```python
from build123d import *

# Parameters (mm, degrees)
CYLINDER004_R     = 7
CYLINDER004_DEPTH = 1
BOX003_W          = 12
BOX003_H          = 21
BOX003_DEPTH      = 19.6
BOX002_W          = 5.7
BOX002_H          = 7.6
BOX002_DEPTH      = 3
BOX001_W          = 35.56
BOX001_H          = 17.78
BOX001_DEPTH      = 10
BOX004_W          = 13.749
BOX004_H          = 12
BOX004_DEPTH      = 4
BOX005_W          = 11.3259
BOX005_H          = 12
BOX005_DEPTH      = 4
CYLINDER005_R     = 3.25
CYLINDER005_DEPTH = 3.5
BOX006_W          = 14.4
BOX006_H          = 9
BOX006_DEPTH      = 11
CYLINDER007_R     = 2
CYLINDER007_DEPTH = 5
CYLINDER006_R     = 2
CYLINDER006_DEPTH = 5
CYLINDER009_R     = 2.5
CYLINDER009_DEPTH = 5
CYLINDER008_R     = 10.9
CYLINDER008_DEPTH = 2.6
BOX007_W          = 18.3
BOX007_H          = 21.8
BOX007_DEPTH      = 24.8
CYLINDER010_R     = 2.5
CYLINDER010_DEPTH = 5
CYLINDER001_R     = 1.8
CYLINDER001_DEPTH = 1.8
CYLINDER002_R     = 1.8
CYLINDER002_DEPTH = 1.8
CYLINDER003_R     = 1.8
CYLINDER003_DEPTH = 1.8
CYLINDER_R        = 1.8
CYLINDER_DEPTH    = 1.8
BOX_W             = 76.2
BOX_H             = 68.58
BOX_DEPTH         = 1.8
FILLET_R          = 3.81
CYLINDER015_R     = 2
CYLINDER015_DEPTH = 5
CYLINDER011_R     = 2
CYLINDER011_DEPTH = 5
CYLINDER012_R     = 2.5
CYLINDER012_DEPTH = 5
CYLINDER014_R     = 10.9
CYLINDER014_DEPTH = 2.6
BOX008_W          = 18.3
BOX008_H          = 21.8
BOX008_DEPTH      = 24.8
CYLINDER013_R     = 2.5
CYLINDER013_DEPTH = 5


with BuildPart() as cylinder004:
    # Cylinder004 → Cylinder004 (new body)
    with BuildSketch(Plane(origin=(0, 50.8, 11.4), x_dir=(0, 0, -1), z_dir=(1, 0, 0))):
        Circle(CYLINDER004_R)
    extrude(amount=CYLINDER004_DEPTH)


with BuildPart() as midi:
    # Box003 → Box003 (new body)
    with BuildSketch(Plane(origin=(0, 40.3, 1.8), x_dir=(1, 0, 0), z_dir=(0, 0, 1))):
        with Locations((6, 10.5)):
            Rectangle(BOX003_W, BOX003_H)
    extrude(amount=BOX003_DEPTH)

    # Cut001: cut Cylinder004
    add(cylinder004.part, mode=Mode.SUBTRACT)


with BuildPart() as cube002:
    # Box002 → Box002 (new body)
    with BuildSketch(Plane(origin=(0, 16.53, 11.8), x_dir=(1, 0, 0), z_dir=(0, 0, 1))):
        with Locations((2.85, 3.8)):
            Rectangle(BOX002_W, BOX002_H)
    extrude(amount=BOX002_DEPTH)


with BuildPart() as obj1:
    # Box001 → Box001 (new body)
    with BuildSketch(Plane(origin=(0, 11.44, 1.8), x_dir=(1, 0, 0), z_dir=(0, 0, 1))):
        with Locations((17.78, 8.89)):
            Rectangle(BOX001_W, BOX001_H)
    extrude(amount=BOX001_DEPTH)

    # Fusion001: union Cube002
    add(cube002.part)


with BuildPart() as obj2:
    # Box004 → Box004 (new body)
    with BuildSketch(Plane(origin=(38.8544, 0, 1.8), x_dir=(1, 0, 0), z_dir=(0, 0, 1))):
        with Locations((6.8745, 6)):
            Rectangle(BOX004_W, BOX004_H)
    extrude(amount=BOX004_DEPTH)


with BuildPart() as obj3:
    # Box005 → Box005 (new body)
    with BuildSketch(Plane(origin=(40.005, 56.58, 1.8), x_dir=(1, 0, 0), z_dir=(0, 0, 1))):
        with Locations((5.66295, 6)):
            Rectangle(BOX005_W, BOX005_H)
    extrude(amount=BOX005_DEPTH)


with BuildPart() as cylinder005:
    # Cylinder005 → Cylinder005 (new body)
    with BuildSketch(Plane(origin=(10.9, 4.5, 8.3), x_dir=(0, 0, -1), z_dir=(1, 0, 0))):
        Circle(CYLINDER005_R)
    extrude(amount=CYLINDER005_DEPTH)


with BuildPart() as dc_jack:
    # Box006 → Box006 (new body)
    with BuildSketch(Plane.XY.offset(1.8)):
        with Locations((7.2, 4.5)):
            Rectangle(BOX006_W, BOX006_H)
    extrude(amount=BOX006_DEPTH)

    # Cut002: cut Cylinder005
    add(cylinder005.part, mode=Mode.SUBTRACT)


with BuildPart() as dc_jack_1:
    # Cut002 placement: moved
    add(dc_jack.part.moved(Location((64.4, 1.85, 0))))


with BuildPart() as cylinder007:
    # Cylinder007 → Cylinder007 (new body)
    with BuildSketch(Plane(origin=(13.3, 20.8, 2.5), x_dir=(0, 0, -1), z_dir=(1, 0, 0))):
        Circle(CYLINDER007_R)
    extrude(amount=CYLINDER007_DEPTH)


with BuildPart() as fusion003:
    # Cylinder006 → Cylinder006 (new body)
    with BuildSketch(Plane(origin=(13.3, 1, 22.3), x_dir=(0, 0, -1), z_dir=(1, 0, 0))):
        Circle(CYLINDER006_R)
    extrude(amount=CYLINDER006_DEPTH)

    # Fusion003: union Cylinder007
    add(cylinder007.part)


with BuildPart() as cylinder009:
    # Cylinder009 → Cylinder009 (new body)
    with BuildSketch(Plane(origin=(13.3, 1, 22.3), x_dir=(0, 0, -1), z_dir=(1, 0, 0))):
        Circle(CYLINDER009_R)
    extrude(amount=CYLINDER009_DEPTH)


with BuildPart() as cylinder008:
    # Cylinder008 → Cylinder008 (new body)
    with BuildSketch(Plane(origin=(18.3, 10.9, 12.4), x_dir=(0, 0, -1), z_dir=(1, 0, 0))):
        Circle(CYLINDER008_R)
    extrude(amount=CYLINDER008_DEPTH)


with BuildPart() as cube005:
    # Box007 → Box007 (new body)
    with BuildSketch(Plane.XY):
        with Locations((9.15, 10.9)):
            Rectangle(BOX007_W, BOX007_H)
    extrude(amount=BOX007_DEPTH)


with BuildPart() as obj4:
    # Cylinder010 → Cylinder010 (new body)
    with BuildSketch(Plane(origin=(13.3, 20.8, 2.5), x_dir=(0, 0, -1), z_dir=(1, 0, 0))):
        Circle(CYLINDER010_R)
    extrude(amount=CYLINDER010_DEPTH)

    # Fusion002: union Cylinder009, Cylinder008, Cube005
    add(cylinder009.part)
    add(cylinder008.part)
    add(cube005.part)

    # Cut003: cut Fusion003
    add(fusion003.part, mode=Mode.SUBTRACT)


with BuildPart() as obj4_1:
    # Cut003 placement: moved
    add(obj4.part.moved(Location((57.9, 15.14, 1.8))))


with BuildPart() as cylinder001:
    # Cylinder001 → Cylinder001 (new body)
    with BuildSketch(Plane(origin=(3.81, 64.77, 0), x_dir=(1, 0, 0), z_dir=(0, 0, 1))):
        Circle(CYLINDER001_R)
    extrude(amount=CYLINDER001_DEPTH)


with BuildPart() as cylinder002:
    # Cylinder002 → Cylinder002 (new body)
    with BuildSketch(Plane(origin=(56.5, 3.81, 0), x_dir=(1, 0, 0), z_dir=(0, 0, 1))):
        Circle(CYLINDER002_R)
    extrude(amount=CYLINDER002_DEPTH)


with BuildPart() as cylinder003:
    # Cylinder003 → Cylinder003 (new body)
    with BuildSketch(Plane(origin=(55.23, 64.77, 0), x_dir=(1, 0, 0), z_dir=(0, 0, 1))):
        Circle(CYLINDER003_R)
    extrude(amount=CYLINDER003_DEPTH)


with BuildPart() as fusion:
    # Cylinder → Cylinder (new body)
    with BuildSketch(Plane(origin=(3.81, 3.81, 0), x_dir=(1, 0, 0), z_dir=(0, 0, 1))):
        Circle(CYLINDER_R)
    extrude(amount=CYLINDER_DEPTH)

    # Fusion: union Cylinder001, Cylinder002, Cylinder003
    add(cylinder001.part)
    add(cylinder002.part)
    add(cylinder003.part)


with BuildPart() as pcb:
    # Box → Box (new body)
    with BuildSketch(Plane.XY):
        with Locations((38.1, 34.29)):
            Rectangle(BOX_W, BOX_H)
    extrude(amount=BOX_DEPTH)

    # Fillet
    fillet_edges = [pcb.edges().sort_by_distance(p)[0] for p in [
        (0, 0, 0.9),
        (0, 68.58, 0.9),
        (76.2, 0, 0.9),
        (76.2, 68.58, 0.9),
    ]]
    fillet(fillet_edges, radius=FILLET_R)

    # Cut: cut Fusion
    add(fusion.part, mode=Mode.SUBTRACT)


with BuildPart() as cylinder015:
    # Cylinder015 → Cylinder015 (new body)
    with BuildSketch(Plane(origin=(13.3, 20.8, 2.5), x_dir=(0, 0, -1), z_dir=(1, 0, 0))):
        Circle(CYLINDER015_R)
    extrude(amount=CYLINDER015_DEPTH)


with BuildPart() as fusion004:
    # Cylinder011 → Cylinder011 (new body)
    with BuildSketch(Plane(origin=(13.3, 1, 22.3), x_dir=(0, 0, -1), z_dir=(1, 0, 0))):
        Circle(CYLINDER011_R)
    extrude(amount=CYLINDER011_DEPTH)

    # Fusion004: union Cylinder015
    add(cylinder015.part)


with BuildPart() as cylinder012:
    # Cylinder012 → Cylinder012 (new body)
    with BuildSketch(Plane(origin=(13.3, 1, 22.3), x_dir=(0, 0, -1), z_dir=(1, 0, 0))):
        Circle(CYLINDER012_R)
    extrude(amount=CYLINDER012_DEPTH)


with BuildPart() as cylinder014:
    # Cylinder014 → Cylinder014 (new body)
    with BuildSketch(Plane(origin=(18.3, 10.9, 12.4), x_dir=(0, 0, -1), z_dir=(1, 0, 0))):
        Circle(CYLINDER014_R)
    extrude(amount=CYLINDER014_DEPTH)


with BuildPart() as cube006:
    # Box008 → Box008 (new body)
    with BuildSketch(Plane.XY):
        with Locations((9.15, 10.9)):
            Rectangle(BOX008_W, BOX008_H)
    extrude(amount=BOX008_DEPTH)


with BuildPart() as device:
    # Cylinder013 → Cylinder013 (new body)
    with BuildSketch(Plane(origin=(13.3, 20.8, 2.5), x_dir=(0, 0, -1), z_dir=(1, 0, 0))):
        Circle(CYLINDER013_R)
    extrude(amount=CYLINDER013_DEPTH)

    # Fusion005: union Cylinder012, Cylinder014, Cube006
    add(cylinder012.part)
    add(cylinder014.part)
    add(cube006.part)

    # Cut004: cut Fusion004
    add(fusion004.part, mode=Mode.SUBTRACT)


with BuildPart() as device_1:
    # Cut004 placement: moved
    add(device.part.moved(Location((57.9, 43.08, 1.8))))

    # Fusion006: union Midi, obj1, obj2, obj3, DC Jack, obj4, PCB
    add(midi.part)
    add(obj1.part)
    add(obj2.part)
    add(obj3.part)
    add(dc_jack_1.part)
    add(obj4_1.part)
    add(pcb.part)


solid = device_1.part
```
Verification items for the finished model (mm, model axes). A direction names the side the tool comes from. Round coordinates to 2 decimals unless told otherwise and drop trailing zeros. Write each loop counter-clockwise with the first axis right and the second up, starting at its lowest first coordinate (ties: lowest second). Pieces come first, ordered by that corner, then holes. Notation, with made-up numbers: (-37.5, 77.25) - (3.5, 77.25) arc R8 ccw to (3.5, 82.25) - close; hole circle Ø5 at (26.5, 78). An arc over 180 degrees is marked (long way). Answer as a JSON object with one key per item and string values. Group by question number.
Q1. Mould release check, pull along Y, two halves, no side actions. Record for faces 6 (the flat face through (71.2, 44, 24)), 7 (the flat face through (3, 16.53, 13)), 8 (the flat face through (37.6, 68.58, 1.6)): released by +Y, released by -Y, zero draft, split by the parting line, or undercut.
Q2. Section check A-A, the plane x = 62.5. Enter the section's corners in (y, z).
Q3. Go/stop test with flat-tipped pins: pin 1 Ø8 at (x, z) = (69, 7.5) entering from +Y; pin 2 Ø6 at (x, z) = (60, 17) entering from -Y; pin 3 Ø2.5 at (y, z) = (5.5, 7.5) entering from -X; pin 4 Ø8 at (y, z) = (44.5, 12) entering from -X. Record where each tip stops, or that it passes through.
Q4. Section check D-D, the plane z = 10.5. Give the number of separate pieces and of enclosed holes in the cut face, plus the area to 3 significant figures.
Q5. Section check B-B, the plane z = 20.5. Enter the section's corners in (x, y).
Q6. Thickness scan on line 1 (Y direction, x = 73.45, z = 24.1); line 2 (Y direction, x = 72.2, z = 4.3); line 3 (Y direction, x = 75, z = 20.75). Record the ranges inside material, lowest first.
Q7. Section check C-C, the plane y = 23. Enter the section's corners in (x, z).
Q8. Tool access check on faces 1 (the flat face through (76.2, 27, 25.4)), 2 (the flat face through (76.2, 35, 2)), 3 (the flat face through (46, 63, 5.8)), 4 (the cylindrical face through (77.48, 21.87, 4.13)), 5 (the cylindrical face through (73.66, 66.38, 4.26)). Record the directions out of +Z, -Z, +X, -X, +Y, -Y that give a thin tool (end or side, any length) a straight path to the whole face; none if there is none.
Found:
{
 "1": {"face 6": "undercut", "face 7": "released by -Y", "face 8": "released by +Y"},
 "2": {"outline": "(0, 0) - (68.58, 0) - (68.58, 1.8) - (64.88, 1.8) - (64.88, 26.6) - (43.08, 26.6) - (43.08, 1.8) - (36.94, 1.8) - (36.94, 26.6) - (15.14, 26.6) - (15.14, 1.8) - (0, 1.8) - close"},
 "3": {"pin 1": "stops at y = 66.38", "pin 2": "stops at y = 15.14", "pin 3": "stops at x = 64.4", "pin 4": "stops at x = 0"},
 "4": {"separate pieces": "5", "enclosed holes": "0", "area": "1,890 mm^2"},
 "5": {"outline": "(0, 40.3) - (12, 40.3) - (12, 61.3) - (0, 61.3) - close; (57.9, 15.14) - (76.2, 15.14) - (76.2, 17.15) - (78.8, 17.15) - (78.8, 34.93) - (76.2, 34.93) - (76.2, 36.94) - (57.9, 36.94) - close; (57.9, 43.08) - (76.2, 43.08) - (76.2, 45.09) - (78.8, 45.09) - (78.8, 62.87) - (76.2, 62.87) - (76.2, 64.88) - (57.9, 64.88) - close"},
 "6": {"line 1": "y = 13.64 to 14.14, 18.14 to 36.94, 41.58 to 42.08, 46.08 to 64.88", "line 2": "y = 1.85 to 10.85, 15.14 to 33.94, 37.94 to 38.44, 43.08 to 61.88, 65.88 to 66.38", "line 3": "y = 15.14 to 36.94, 43.08 to 64.88"},
 "7": {"outline": "(0, 0) - (76.2, 0) - (76.2, 3.73) - (78.8, 3.73) - (78.8, 24.67) - (76.2, 24.67) - (76.2, 26.6) - (57.9, 26.6) - (57.9, 1.8) - (35.56, 1.8) - (35.56, 11.8) - (5.7, 11.8) - (5.7, 14.8) - (0, 14.8) - close"},
 "8": {"face 1": "+Z, +X", "face 2": "-Z, +X", "face 3": "+Z, +Y, -Y", "face 4": "+X", "face 5": "+X, +Y"}
}
